from build123d import *

# Parameters (mm, degrees)
SKETCH1_R           = 2.38125
BOSS_EXTRUDE1_DEPTH = 3.175
BOSS_EXTRUDE2_DEPTH = 3.175


with BuildPart() as part:
    # Sketch1 → Boss-Extrude1 (new body)
    with BuildSketch(Plane.XY):
        with BuildLine():
            Line((-19.05, 0), (0, 0))
            Line((0, 0), (0, 3.175))
            Line((0, 3.175), (-12.7, 3.175))
            add(Edge.make_bspline(
                [(-19.05, 0), (-13.112033971, -2.27730223), (-5.155795632, -3.204594962), (8.217288269, -6.774378233), (12.030948412, 0.931903495), (12.931224231, 8.259301282), (4.816413804, 15.369954974), (-3.592277072, 7.785567441), (-9.215384474, 5.719027598), (-12.7, 3.175)],
                knots=[0, 0, 0, 0, 0.256909303, 0.405237787, 0.477393103, 0.59131784, 0.708774719, 0.830232282, 1, 1, 1, 1], degree=3))
        make_face()
        with Locations((5.048367475, 8.51005191)):
            Circle(SKETCH1_R, mode=Mode.SUBTRACT)
    extrude(amount=BOSS_EXTRUDE1_DEPTH)

    # Sketch2 → Boss-Extrude2 (add)
    with BuildSketch(Plane.XY.offset(3.175)):
        with BuildLine():
            add(Edge.make_bspline(
                [(4.988150959, 13.056659727), (9.718743656, 12.859855216), (14.559374774, 12.389270948), (19.04312554, 10.761627981)],
                knots=[0, 0, 0, 0, 1, 1, 1, 1], degree=3))
            Line((4.988150959, 13.056659727), (8.479749464, 10.133745789))
            Line((8.479749464, 10.133745789), (7.569273367, -4.93526217))
            add(Edge.make_bspline(
                [(7.569273367, -4.93526217), (10.177388397, -3.973098163), (15.151025201, -1.968746735), (20.532585299, -4.307476576), (22.21812554, -1.938372019)],
                knots=[0, 0, 0, 0, 0.552836204, 1, 1, 1, 1], degree=3))
            Line((22.21812554, -1.938372019), (9.51812554, -1.938372019))
            Line((9.51812554, -1.938372019), (9.51812554, 10.761627981))
            Line((9.51812554, 10.761627981), (19.04312554, 10.761627981))
        make_face()
        Polygon((19.04312554, 4.411627981), (19.04312554, 10.761627981), (9.51812554, 10.761627981), (9.51812554, -1.938372019), (22.21812554, -1.938372019), (22.21812554, 4.411627981), align=None)
    extrude(amount=-BOSS_EXTRUDE2_DEPTH)


solid = part.part
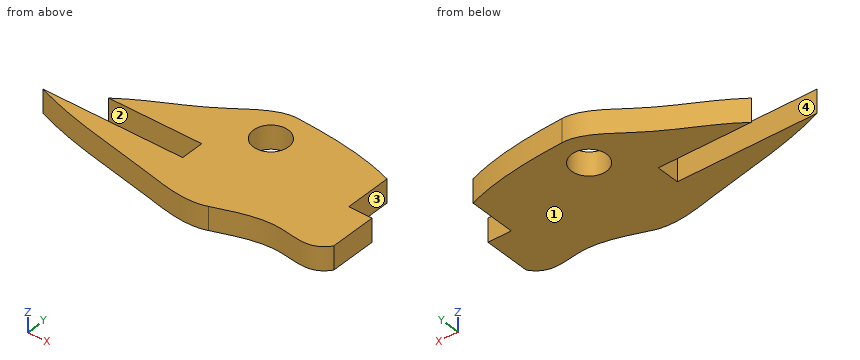
CAD build for the part. Positions are in the model's coordinates, mm. Face numbers are marked on the shaded views. A direction names the side the tool comes from. Coordinates: 2 decimals unless noted, no trailing zeros. Loops run counter-clockwise (first coordinate to the right, second up) from the corner with the lowest first, then second, coordinate; pieces in that order, holes last. Notation, with made-up numbers: (42, 46.25) - (90, 46.25) arc R15 cw to (90, 74.25) - close; hole circle Ø7 at (52, 2.5). An arc over 180 degrees is marked (long way). Use one line per item in the form item = value. Start each with the question number.
1) Tool access for the marked faces 1 and 2: list every direction of +Z, -Z, +X, -X, +Y, -Y with a clear straight run to the whole face (end or side of a thin tool).
2) Flat gauge pins, fed straight in: pin 1 (4 mm diameter, centred on x = 16.5, y = 0.5, fed in from -Z); pin 2 (1 mm diameter, centred on x = -12, z = 2, fed in from +Y); pin 3 (1.6 mm diameter, centred on x = 20, z = 1, fed in from +Y); pin 4 (1 mm diameter, centred on y = 6.5, z = 1, fed in from +X). Where does each tip first touch, or does it go through?
3) Drill centre lines: L1, parallel to X at y = 1.5, z = 2.4; L2, parallel to Y at x = -10, z = 1.3 (3 decimals); L3, parallel to X at y = 9, z = 1.9. Where is each one in solid material? Low to high. Write a range as from..to.
4) Two-plate mould, pull along Y, no slides. Class the marked faces 3 and 4: +Y half, -Y half, draft (parallel to the pull), parting line (faces both ways), or undercut.
5) Band-saw the part on A-A (y = 2.5). Give the cut face in (x, z) (3 decimals).
Check values:
q1.face_1 = -Z, +X, -X, +Y, -Y
q1.face_2 = +Z, -Z, -X
q2.pin_1 = 0
q2.pin_2 = 4.01
q2.pin_3 = 4.41
q2.pin_4 = 19.04
q3.L1 = 0..22.22
q3.L2 = -2.58..0, 3.175..4.942
q3.L3 = -2.92..2.72, 7.38..19.04
q4.face_3 = draft
q4.face_4 = undercut
q5.outline = (0, 0) - (22.218, 0) - (22.218, 3.175) - (0, 3.175) - close
